from build123d import *

# Parameters (mm, degrees)
SKETCH1_R               = 3.2639
BOSS_EXTRUDE1_DEPTH     = 2.38125
F_1_4_CLEARANCE_HOLE1_D = 7.14248


with BuildPart() as part:
    # Sketch1 → Boss-Extrude1 (new, symmetric)
    with BuildSketch(Plane.XY):
        Polygon((0, 0), (0, 76.2), (25.4, 76.2), (76.2, 25.4), (76.2, 0), align=None)
        with Locations(Location((12.7, 12.7, 0), (0, 0, 180))):
            Circle(SKETCH1_R, mode=Mode.SUBTRACT)
        with Locations(Location((38.1, 12.7, 0), (0, 0, 180))):
            Circle(SKETCH1_R, mode=Mode.SUBTRACT)
        with Locations(Location((63.5, 12.7, 0), (0, 0, 180))):
            Circle(SKETCH1_R, mode=Mode.SUBTRACT)
        with Locations(Location((12.7, 38.1, 0), (0, 0, 180))):
            Circle(SKETCH1_R, mode=Mode.SUBTRACT)
        with Locations(Location((12.7, 63.5, 0), (0, 0, 180))):
            Circle(SKETCH1_R, mode=Mode.SUBTRACT)
    extrude(amount=BOSS_EXTRUDE1_DEPTH, both=True)

    # 1/4 Clearance Hole1 (through all)
    with Locations(Plane.XY.offset(2.38125)):
        with Locations((12.7, 63.5), (12.7, 38.1), (12.7, 12.7), (38.1, 12.7), (63.5, 12.7)):
            Hole(F_1_4_CLEARANCE_HOLE1_D / 2)


solid = part.part
Verification items for the finished model (mm, model axes). Give positions to 0.01 mm unless a question says otherwise; leave off trailing zeros. Loops run counter-clockwise (first coordinate to the right, second up) from the corner with the lowest first, then second, coordinate; pieces in that order, holes last.
1. Cross-section at A-A on x = 12.7. Record the cut outline in (y, z), and give its area (3 significant figures).
Derived:
outline: (0, -2.38) - (9.13, -2.38) - (9.13, 2.38) - (0, 2.38) - close; (16.27, -2.38) - (34.53, -2.38) - (34.53, 2.38) - (16.27, 2.38) - close; (41.67, -2.38) - (59.93, -2.38) - (59.93, 2.38) - (41.67, 2.38) - close; (67.07, -2.38) - (76.2, -2.38) - (76.2, 2.38) - (67.07, 2.38) - close
area: 261 mm2
2. Material ranges on probe 1 along Y at (x, z) = (12.7, 0.55); probe 2 along Y at (x, z) = (63.5, -1.95); probe 3 along Y at (x, z) = (36, -0.25), recorded low to high.
Derived:
probe 1: y = 0 to 9.13, 16.27 to 34.53, 41.67 to 59.93, 67.07 to 76.2
probe 2: y = 0 to 9.13, 16.27 to 38.1
probe 3: y = 0 to 9.81, 15.59 to 65.6
3. Go/stop test with a flat-tipped pin: P1, Ø1, axis at x = 50.5, z = -1.5, coming from the +Y side. Record where the tip stops, or that it passes through.
Derived:
P1: stops at y = 51.6
4. Release check for a two-part mould opening along X. For faces 1 (the flat face through (50.4, 51.2, 0)), 2 (the cylindrical face through (13.16, 67.04, -0.03)), 3 (the cylindrical face through (41.668, 12.857, -0.033)), 4 (the flat face through (30, 30, -2.381)) record: +X half, -X half, draft (parallel to the pull), parting line (faces both ways), or undercut.
Derived:
face 1: +X half
face 2: undercut
face 3: undercut
face 4: draft
5. Cross-section at D-D on z = -0.5. Record the cut outline in (x, y).
Derived:
outline: (0, 0) - (76.2, 0) - (76.2, 25.4) - (25.4, 76.2) - (0, 76.2) - close; hole circle Ø7.14 at (12.7, 12.7); hole circle Ø7.14 at (12.7, 38.1); hole circle Ø7.14 at (12.7, 63.5); hole circle Ø7.14 at (38.1, 12.7); hole circle Ø7.14 at (63.5, 12.7)
6. Cross-section at B-B on y = 38.1. Record the cut outline in (x, z), and give its area (3 significant figures).
Derived:
outline: (0, -2.38) - (9.13, -2.38) - (9.13, 2.38) - (0, 2.38) - close; (16.27, -2.38) - (63.5, -2.38) - (63.5, 2.38) - (16.27, 2.38) - close
area: 268 mm2
